Part model, mm, in its own coordinate system. A direction names the side the tool comes from. Coordinates: 2 decimals unless noted, no trailing zeros. Loops run counter-clockwise (first coordinate to the right, second up) from the corner with the lowest first, then second, coordinate; pieces in that order, holes last. Notation, with made-up numbers: (85.25, -39.75) -> (99.25, -39.75) arc R10 cw to (99.25, -28.75) -> close; hole circle Ø5 at (81.5, 9.5). An arc over 180 degrees is marked (long way). Use one line per item in the form item = value. Start each with the question number.
(1) Drill centre lines: L1, parallel to Z at x = -16, y = 19; L2, parallel to X at y = 3, z = 10; L3, parallel to Y at x = -24, z = 28.5. Where is each one in solid material? Low to high. Write a range as [from, to].
(2) Pin check, flat tips, straight feed: P1, Ø12, axis at x = -4, z = 14.5, coming from the -Y side; P2, Ø1, axis at x = -32.5, y = 25.5, coming from the -Z side; P3, Ø15, axis at y = 11, z = 11, coming from the -X side; P4, Ø6, axis at x = -8.5, y = 18, coming from the +Z side. Stop position of each tip, or through.
(3) Mould opens along Y. For faces 1 (the flat face through (-19, 61.773, 15)), 2 (the flat face through (-19, 16, 29.896)), 3 (the flat face through (-14.1, 32.36, 28.4)) say: +Y half, -Y half, draft (parallel to the pull), parting line (faces both ways), or undercut.
(4) Band-saw the part on B-B on y = 43.5. Give the cut face in (x, z), then the cut area to 3 significant figures.
(5) Band-saw the part on A-A on y = 26.5. Give the cut face in (x, z), then the cut area to 3 significant figures.
(6) 3-axis set-ups, long thin cutter, end or side, ignore diameter. For faces 4 (the flat face through (0, 16, 15)), 5 (the flat face through (-36.957, 16, 15)), 6 (the cylindrical face through (-32.435, 44.519, 15.562)), 7 (the flat face through (-18, 0, 15)), 8 (the flat face through (-18, 16, 0)): which of +Z, -Z, +X, -X, +Y, -Y reach the whole face in a straight line?
Autodesk Inventor part; units mm, degrees
ref_plane "YZ Plane" through (0, 0, 0) normal (1, 0, 0) x (0, 1, 0)
ref_plane "XZ Plane" through (0, 0, 0) normal (0, 1, 0) x (-1, 0, 0)
ref_plane "XY Plane" through (0, 0, 0) normal (0, 0, 1) x (1, 0, 0)
sketch "Sketch1" plane through (0, 0, 0) normal (0, 1, 0) x (-1, 0, 0)
  line L0 (0, 0) -> (36.957, 0)
  line L1 (36.957, 0) -> (36.957, 29.8958)
  line L2 (36.957, 29.8958) -> (0, 29.8958)
  line L3 (0, 29.8958) -> (0, 0)
  dimension "d0" = 36.957
  dimension "d1" = 29.8958
extrude "Extrusion1" add sketch "Sketch1" along normal blind 32.3596
sketch "Sketch2" plane through (0, 32.3596, 0) normal (0, 1, 0) x (1, 0, 0)
  circle A0 centre (-18.4785, -14.9479) radius 13.97
  dimension "d4" = 27.94
extrude "Extrusion2" add sketch "Sketch2" along normal blind 24.6634
sketch "Sketch3" plane through (-18.4785, 57.023, 14.9479) normal (0, 1, 0) x (1, 0, 0)
  circle A0 centre (0, 0) radius 13.97
  point P0 (18.4785, 14.9479)
sketch "Sketch4" plane through (-18.4785, 57.023, 14.9479) normal (0, 1, 0) x (1, 0, 0)
  circle A0 centre (0, 0) radius 13.97
  circle A1 centre (0, 0) radius 19.8628
  point P0 (18.4785, 14.9479)
  dimension "d7" = 39.7256
extrude "Extrusion3" add sketch "Sketch4" along normal blind 4.7498 contours A0 | A1
fillet "Fillet1" radius 7.62 1 edges at (-38.3413, 61.7728, 14.9479)
properties part number "Button"
A:
q1.L1 = [0, 29.9]
q1.L2 = [-36.96, 0]
q1.L3 = [0, 32.36], [57.02, 61.55]
q2.P1 = 0
q2.P2 = 0
q2.P3 = -36.96
q2.P4 = 29.9
q3.face_1 = +Y half
q3.face_2 = draft
q3.face_3 = undercut
q4.outline = circle Ø27.94 at (-18.48, 14.95)
q4.area = 613 mm²
q5.outline = (-36.96, 0) -> (0, 0) -> (0, 29.9) -> (-36.96, 29.9) -> close
q5.area = 1,100 mm²
q6.face_4 = +Z, -Z, +X, -Y
q6.face_5 = +Z, -Z, -X, -Y
q6.face_6 = none
q6.face_7 = +Z, -Z, +X, -X, -Y
q6.face_8 = -Z, +X, -X, -Y
